Autodesk Inventor part; units mm, degrees
ref_plane "YZ Plane" through (0, 0, 0) normal (1, 0, 0) x (0, 1, 0)
ref_plane "XZ Plane" through (0, 0, 0) normal (0, 1, 0) x (-1, 0, 0)
ref_plane "XY Plane" through (0, 0, 0) normal (0, 0, 1) x (1, 0, 0)
sketch "Sketch1" plane through (0, 0, 0) normal (0, 1, 0) x (-1, 0, 0)
  line L0 (-8.3746, 16.5585) -> (42.4254, 16.5585)
  line L1 (42.4254, 16.5585) -> (42.4254, 14.0185)
  line L2 (42.4254, 14.0185) -> (33.5354, 14.0185)
  line L3 (33.5354, 14.0185) -> (33.5354, -11.3815)
  line L4 (33.5354, -11.3815) -> (42.4254, -11.3815)
  line L5 (42.4254, -11.3815) -> (42.4254, -13.9215)
  line L6 (42.4254, -13.9215) -> (-8.3746, -13.9215)
  line L7 (-8.3746, 16.5585) -> (-8.3746, 14.0185)
  line L8 (-8.3746, 14.0185) -> (23.3754, 14.0185)
  line L9 (23.3754, 14.0185) -> (23.3754, -11.3815)
  line L10 (23.3754, -11.3815) -> (-8.3746, -11.3815)
  line L11 (-8.3746, -11.3815) -> (-8.3746, -13.9215)
  point P0 (0, 0)
  dimension "d0" = 30.48
  dimension "d1" = 2.54
  dimension "d2" = 2.54
  dimension "d4" = 2.54
  dimension "d5" = 2.54
  dimension "d6" = 8.89
  dimension "d7" = 50.8
  dimension "d8" = 31.75
extrude "Extrusion1" add sketch "Sketch1" along normal blind 25.4
sketch "Sketch4" plane through (8.3746, 0, -13.9215) normal (0, 0, -1) x (-1, 0, 0)
  line L0 (50.8, 0) -> (0, 0)
  line L1 (50.8, 0) -> (50.8, 25.4)
  line L2 (0, 25.4) -> (50.8, 25.4)
  line L3 (50.8, 25.4) -> (41.91, 25.4)
  line L4 (41.91, 25.4) -> (41.91, 0)
  line L5 (41.91, 0) -> (50.8, 0)
  line L6 (50.8, 0) -> (50.8, 25.4)
  point P0 (8.3746, 0)
  dimension "d56" = 8.89
extrude "Extrusion3" add sketch "Sketch4" along normal blind 11.43
sketch "Sketch5" plane through (-42.4254, 0, 16.5585) normal (0, 0, 1) x (1, 0, 0)
  line L0 (50.8, 0) -> (50.8, 25.4)
  line L1 (50.8, 0) -> (0, 0)
  point P0 (40.64, 12.7)
  dimension "d11" = 10.16
  dimension "d12" = 12.7
hole "Hole1" at (-1.7854, 12.7, 16.5585) direction (0, 0, -1) diameter 9.779 end through all
sketch "Sketch6" plane through (-42.4254, 0, 16.5585) normal (0, 0, 1) x (1, 0, 0)
  line L0 (0, 0) -> (0, 25.4)
  line L1 (50.8, 0) -> (0, 0)
  point P0 (4, 4)
  dimension "d20" = 4
  dimension "d21" = 4
hole "Hole2" at (-38.4254, 4, 16.5585) direction (0, 0, -1) diameter 4.5 end through all
sketch "Sketch2" plane through (-42.4254, 0, 16.5585) normal (0, 0, 1) x (1, 0, 0)
  circle A0 centre (40.64, 12.7) radius 4.8895
  line L0 (40.64, 22.225) -> (40.64, 3.175) construction
  circle A1 centre (40.64, 12.7) radius 4.8895 construction
  line L1 (40.64, 12.7) -> (33.9048, 19.4352) construction
  line L2 (40.64, 12.7) -> (33.9048, 5.9648) construction
  line L3 (40.64, 12.7) -> (47.3752, 5.9648) construction
  line L4 (40.64, 12.7) -> (47.3752, 19.4352) construction
  point P0 (42.4254, 0)
  dimension "d29" = 9.525
  dimension "d30" = 0
  dimension "d33" = 360
  dimension "d60" = 45
  dimension "d63" = 360
hole "Hole3" at (-1.7854, 3.175, 16.5585) at (-1.7854, 22.225, 16.5585) at (-8.5206, 5.9648, 16.5585) at (-8.5206, 19.4352, 16.5585) at (4.9498, 19.4352, 16.5585) at (4.9498, 5.9648, 16.5585) direction (0, 0, -1) diameter 2.794 end through all
hole "Hole4" at (-33.5354, 22.1488, 1.9535) direction (1, 0, 0) diameter 3.81 end through all
sketch "Sketch7" plane through (8.3746, 0, -25.3515) normal (0, 0, -1) x (-1, 0, 0)
  circle A0 centre (46.355, 19.1807) radius 1.524
  circle A1 centre (46.355, 12.5767) radius 1.524
  line L0 (50.8, 0) -> (50.8, 25.4) construction
  line L1 (41.91, 25.4) -> (41.91, 0) construction
  line L2 (50.8, 25.4) -> (41.91, 25.4) construction
  point P0 (8.3746, 0)
  point P1 (50.8, 3.175)
  dimension "d65" = 3.048
  dimension "d66" = 3.048
  dimension "d67" = 6.604
  dimension "d68" = 8.89
  dimension "d69" = 4.445
  dimension "d70" = 4.445
  dimension "d71" = 6.2193
extrude "Extrusion4" cut sketch "Sketch7" against normal up to surface (13.97 mm away)
ref_plane "Work Plane2" through (-23.3754, 0, 10.8435) normal (1, 0, 0) x (0, 0, -1)
sketch "Sketch8" plane through (-23.3754, 0, 10.8435) normal (1, 0, 0) x (0, 0, -1)
  line L0 (24.765, 0) -> (22.225, 0)
  line L1 (-3.175, 0) -> (-5.715, 0)
  line L2 (22.225, 0) -> (-3.175, 0)
  line L3 (-3.175, 0) -> (-3.175, 12.7)
  line L4 (-3.175, 0) -> (-3.175, 25.4)
  line L5 (-3.175, 12.7) -> (22.225, 12.7)
  line L6 (22.225, 0) -> (-3.175, 0)
  line L7 (22.225, 12.7) -> (22.225, 0)
  point P0 (10.8435, 0)
extrude "Extrusion5" cut sketch "Sketch8" against normal through all
sketch "Sketch10" plane through (0, 25.4, 0) normal (0, 1, 0) x (1, 0, 0)
  line L0 (-42.4254, 25.3515) -> (-33.5354, 25.3515)
  line L1 (-33.5354, 25.3515) -> (-24.6454, 25.3515)
  line L2 (-24.6454, 25.3515) -> (-24.6454, 13.9215)
  line L3 (8.3746, 13.9215) -> (-33.5354, 13.9215)
  line L4 (-33.5354, 13.9215) -> (-33.5354, 25.3515)
  line L5 (-33.5354, 13.9215) -> (-24.6454, 13.9215)
  line L6 (-33.5354, 13.9215) -> (-33.5354, 25.3515)
  point P0 (0, 0)
  dimension "d76" = 8.89
extrude "Extrusion6" add sketch "Sketch10" against normal blind 25.4
sketch "Sketch11" plane through (0, 0, 0) normal (0, -1, 0) x (1, 0, 0)
  line L0 (-42.4254, -22.8115) -> (-33.5354, -22.8115)
  line L1 (-23.3754, -11.3815) -> (-33.5354, -11.3815)
  line L2 (-33.5354, -22.8115) -> (-33.5354, -11.3815)
  line L3 (-42.4254, -11.3815) -> (-33.5354, -11.3815)
  line L4 (-33.5354, -11.3815) -> (-42.4254, -11.3815)
  line L5 (-42.4254, -11.3815) -> (-42.4254, -22.8115)
  point P0 (0, 0)
  point P1 (-42.4254, -25.3515)
  dimension "d79" = 2.54
extrude "Extrusion7" cut sketch "Sketch11" against normal through all
equation "\"d2\" = d1"
equation "\"d4\" = d1"
equation "\"d5\" = d1"
equation "\"d69\" = 0.5 * d68"
equation "\"d70\" = 0.5 * d68"
properties part number "Odometry_Holder for metal drivetrain"
Design review of the part built by this model. Coordinates are the model's own, in mm. A direction names the side the tool comes from. Coordinates: 2 decimals unless noted, no trailing zeros. Write each loop counter-clockwise with the first axis right and the second up, starting at its lowest first coordinate (ties: lowest second). Pieces come first, ordered by that corner, then holes. Notation, with made-up numbers: M 18,80 L 68,80 A26 ccw 68,94 Z; hole C 87.5,-10 d11. An arc over 180 degrees is marked long. Answer as a JSON object with one key per item and string values.
Item 1: Wall thickness on probe 1 along Z at (x, y) = (5.5, 24); probe 2 along Z at (x, y) = (-29.5, 4.5); probe 3 along X at (y, z) = (4, -24.75): over which ranges is each line inside the solid? List them lowest first.
Outcome:
{"probe 1": "-13.92 to -11.38, 14.02 to 16.56", "probe 2": "-25.35 to -11.38, 14.02 to 16.56", "probe 3": "-42.43 to -40.68, -36.18 to -24.65"}
Item 2: Draft analysis for pull direction X (two halves, no side actions). For faces 4 (the cylindrical face through (-9.465, 6.994, 15.271)), 5 (the flat face through (-34, 13, -25.352)), 6 (the flat face through (-42.425, 13, 15)), state which applies: pulls with the +X half, pulls with the -X half, needs draft (parallel to the pull), parting line crosses it, or undercut.
Outcome:
{"face 4": "undercut", "face 5": "needs draft", "face 6": "pulls with the -X half"}
Item 3: Machinability: for faces 1 (the cylindrical face through (-9.699, 18.684, -12.669)), 2 (the flat face through (-33.535, 15, -8)), 3 (the cylindrical face through (-36.77, 11.65, -24.1)), which of the approach directions +Z, -Z, +X, -X, +Y, -Y give a long, thin tool a straight path to every point of the face, cutting with its end or side? Answer none if there is none.
Outcome:
{"face 1": "+Z, -Z", "face 2": "-X, +Y, -Y", "face 3": "-Z"}
Item 4: Insertion check: pin 1 Ø4 at (y, z) = (17.5, 0.5) entering from +X; pin 2 Ø1.5 at (y, z) = (17.5, -15.5) entering from +X; pin 3 Ø8 at (x, z) = (-29, 5.5) entering from -Y. Each pin has a flat end and moves straight along its axis. Give the tip position at first contact, or say it passes through.
Outcome:
{"pin 1": "x = -23.38", "pin 2": "x = -24.65", "pin 3": "y = 12.7"}
Item 5: Add section A-A, the plane x = -11. Give the boundary of the cut face in (y, z).
Outcome:
{"outline": "M 0,-13.92 L 25.4,-13.92 L 25.4,-11.38 L 0,-11.38 Z; M 0,14.02 L 25.4,14.02 L 25.4,16.56 L 0,16.56 Z"}
Item 6: Add section B-B, the plane z = 3. Give the boundary of the cut face in (x, y), and give its area (3 significant figures).
Outcome:
{"outline": "M -33.54,12.7 L -23.38,12.7 L -23.38,20.56 L -33.54,20.56 Z; M -33.54,23.74 L -23.38,23.74 L -23.38,25.4 L -33.54,25.4 Z", "area": "96.7 mm²"}
Item 7: Add section C-C, the plane y = 4. Give the boundary of the cut face in (x, z).
Outcome:
{"outline": "M -42.43,-25.35 L -40.68,-25.35 L -40.68,-22.81 L -42.43,-22.81 Z; M -42.43,14.02 L -40.68,14.02 L -40.68,16.56 L -42.43,16.56 Z; M -36.18,-25.35 L -24.65,-25.35 L -24.65,-13.92 L -2.91,-13.92 L -2.91,-11.38 L -33.54,-11.38 L -33.54,-22.81 L -36.18,-22.81 Z; M -36.18,14.02 L -2.91,14.02 L -2.91,16.56 L -36.18,16.56 Z; M -0.66,-13.92 L 8.37,-13.92 L 8.37,-11.38 L -0.66,-11.38 Z; M -0.66,14.02 L 8.37,14.02 L 8.37,16.56 L -0.66,16.56 Z"}
Item 8: Add section D-D, the plane x = -25.5. Give the boundary of the cut face in (y, z) (1 decimal), and give its area (3 significant figures).
Outcome:
{"outline": "M 0,-25.4 L 25.4,-25.4 L 25.4,16.6 L 0,16.6 L 0,14 L 12.7,14 L 12.7,-11.4 L 0,-11.4 Z; hole C 22.1,2 d3.8", "area": "731 mm²"}
